Geometry: see drawing. Coordinates: mm, zero at the bounding-box minimum. Give positions to 0.01 mm unless a question says otherwise; leave off trailing zeros. Order: outer loops, then holes, each group sorted by start corner. A loop starts at its lowest first (then second) coordinate and runs counter-clockwise, first axis right, second up. Notation, with made-up numbers: M -4,49.5 L 51,49.5 A20 ccw 51,55.5 Z; hole C 41,-9 d4. An arc over 180 degrees is marked long. Use a Markdown table: item, result.
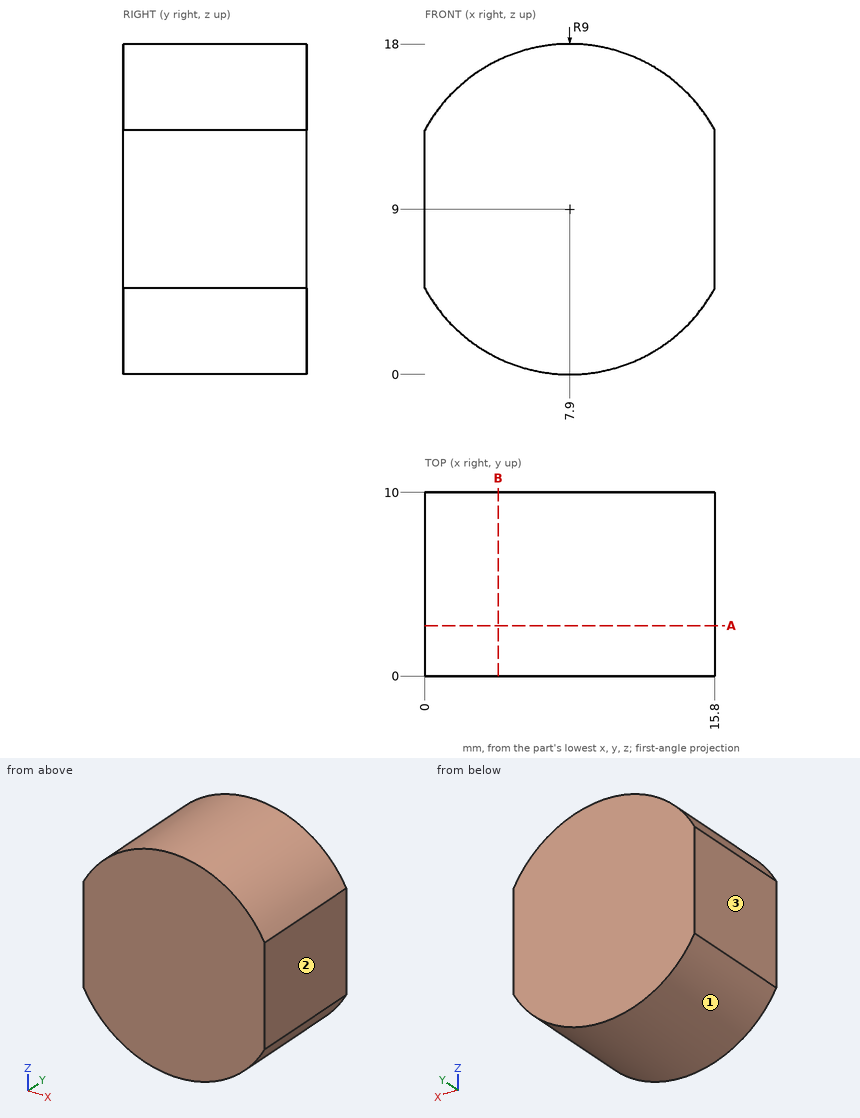
1) Mould query, pull axis X, two halves, no side actions, for the marked faces 1, 2 and 3. Classes: released by +X, released by -X, zero draft, split by the parting line, or undercut.
Response values:
| item | result |
|---|---|
| face 1 | split by the parting line |
| face 2 | released by +X |
| face 3 | released by -X |
2) Cut plane A-A on y = 2.75. Return loops of the section in (x, z).
Response values:
| item | result |
|---|---|
| outline | M 0,4.69 A9 ccw 15.8,4.69 L 15.8,13.31 A9 ccw 0,13.31 Z |
3) Cut plane B-B on x = 4. Return loops of the section in (y, z), and give its area (3 significant figures).
Response values:
| item | result |
|---|---|
| outline | M 0,0.89 L 10,0.89 L 10,17.11 L 0,17.11 Z |
| area | 162 mm² |
4) First-contact query: pin 1 Ø1.5 at (y, z) = (5.5, 3) entering from -X; pin 2 Ø1 at (y, z) = (2.5, 3) entering from +X; pin 3 Ø5 at (x, y) = (3, 8) entering from +Z. Flat tips, straight axial feed; report the tip coordinate or a pass-through.
Response values:
| item | result |
|---|---|
| pin 1 | stops at x = 0.59 |
| pin 2 | stops at x = 15.02 |
| pin 3 | stops at z = 17.67 |
5) Material intervals for line 1 (Z direction, x = 13.25, y = 3.75); line 2 (Z direction, x = 5.5, y = 8.25); line 3 (X direction, y = 8.5, z = 15.75), sorted ascending. Write a range as from..to.
Response values:
| item | result |
|---|---|
| line 1 | z = 1.76..16.24 |
| line 2 | z = 0.33..17.67 |
| line 3 | x = 1.95..13.85 |
